```python
from build123d import *

# Parameters (mm, degrees)
SKETCH_1_R               = 39.75
EXTRUDE_1_DEPTH          = 10
SKETCH_2_R               = 18.25
CUT_EXTRUDE_1_DEPTH      = 4
SKETCH_3_R               = 11.5
CUT_EXTRUDE_2_DEPTH      = 2
SKETCH_4_R               = 1.5
CUT_EXTRUDE_3_DEPTH      = 6
SKETCH_5_R               = 3
CUT_EXTRUDE_4_DEPTH      = 2
SKETCH_7_R               = 2.65
CUT_EXTRUDE_5_DEPTH      = 8
PATTERN_CIRCULAR_1_COUNT = 2
PATTERN_CIRCULAR_1_ANGLE = 25
F_1_THE_OTHER_WAY_COUNT  = 2
F_1_THE_OTHER_WAY_ANGLE  = 25
MIRROR_1_COPY_1_SKETCH_R = 2.65
MIRROR_1_COPY_1_DEPTH    = 8
MIRROR_1_COPY_2_SKETCH_R = 2.65
MIRROR_1_COPY_2_DEPTH    = 8
SKETCH_8_R               = 8
CUT_EXTRUDE_6_DEPTH      = 4
SKETCH_9_R               = 2.65
CUT_EXTRUDE_7_DEPTH      = 8
PATTERN_CIRCULAR_2_COUNT = 2
EXTRUDE_START            = 5
SKETCH_10_R              = 23.25
SKETCH_10_R_2            = 18.25
EXTRUDE_2_DEPTH          = 5
CUT_EXTRUDE_START        = -10
CUT_EXTRUDE_8_DEPTH      = 10
FILLET_1_R               = 1


# Read off the part's stored shape, not the designer's step: Вырез-Вытянуть8
with BuildPart() as part:
    # Эскиз1 → Бобышка-Вытянуть1 (new body)
    with BuildSketch(Plane.XY):
        Circle(SKETCH_1_R)
    extrude(amount=EXTRUDE_1_DEPTH)

    # Эскиз2 → Вырез-Вытянуть1 (cut)
    with BuildSketch(Plane.XY.offset(10)):
        Circle(SKETCH_2_R)
    extrude(amount=-CUT_EXTRUDE_1_DEPTH, mode=Mode.SUBTRACT)

    # Эскиз3 → Вырез-Вытянуть2 (cut)
    with BuildSketch(Plane.XY.offset(6)):
        Circle(SKETCH_3_R)
    extrude(amount=-CUT_EXTRUDE_2_DEPTH, mode=Mode.SUBTRACT)

    # Эскиз4 → Вырез-Вытянуть3 (cut)
    with BuildSketch(Plane.XY.offset(6)):
        with Locations((-9.899494937, 9.899494937)):
            Circle(SKETCH_4_R)
        with Locations((9.899494937, 9.899494937)):
            Circle(SKETCH_4_R)
        with Locations((9.899494937, -9.899494937)):
            Circle(SKETCH_4_R)
        with Locations((-9.899494937, -9.899494937)):
            Circle(SKETCH_4_R)
    extrude(amount=-CUT_EXTRUDE_3_DEPTH, mode=Mode.SUBTRACT)

    # Эскиз5 → Вырез-Вытянуть4 (cut)
    with BuildSketch(Plane(origin=(0, 0, 0), x_dir=(-1, 0, 0), z_dir=(0, 0, -1))):
        with Locations((-9.899494937, 9.899494937)):
            Circle(SKETCH_5_R)
        with Locations((9.899494937, 9.899494937)):
            Circle(SKETCH_5_R)
        with Locations((9.899494937, -9.899494937)):
            Circle(SKETCH_5_R)
        with Locations((-9.899494937, -9.899494937)):
            Circle(SKETCH_5_R)
    extrude(amount=-CUT_EXTRUDE_4_DEPTH, mode=Mode.SUBTRACT)

    # Эскиз7 → Вырез-Вытянуть5 (cut)
    with BuildSketch(Plane(origin=(0, 39.75, 0), x_dir=(0, 0, -1), z_dir=(0, 1, 0))):
        with Locations(Location((-5, 0, 0), (0, 0, 90))):
            Circle(SKETCH_7_R)
    cut_extrude_5 = extrude(amount=-CUT_EXTRUDE_5_DEPTH, mode=Mode.SUBTRACT)

    # Круговой массив1: Вырез-Вытянуть5 ×2 about axis
    pattern_circular_1_axis = Axis((0, 0, 10), (0, 0, -1))
    for i in range(1, PATTERN_CIRCULAR_1_COUNT):
        add(cut_extrude_5.rotate(pattern_circular_1_axis, i * PATTERN_CIRCULAR_1_ANGLE / (PATTERN_CIRCULAR_1_COUNT - 1)), mode=Mode.SUBTRACT)

    # 1 the other way: Вырез-Вытянуть5 ×2 about axis
    f_1_the_other_way_axis = Axis((0, 0, 10), (0, 0, 1))
    for i in range(1, F_1_THE_OTHER_WAY_COUNT):
        add(cut_extrude_5.rotate(f_1_the_other_way_axis, i * F_1_THE_OTHER_WAY_ANGLE / (F_1_THE_OTHER_WAY_COUNT - 1)), mode=Mode.SUBTRACT)

    # Зеркальное отражение1: Вырез-Вытянуть5 across plane
    add(cut_extrude_5.mirror(Plane.ZX), mode=Mode.SUBTRACT)

    # Зеркальное отражение1 copy 1 sketch → Зеркальное отражение1 copy 1 (cut)
    with BuildSketch(Plane(origin=(16.799075904, -36.025734535, 0), x_dir=(0, 0, -1), z_dir=(0.4226182617407035, -0.906307787036648, 0))):
        with Locations((-5, 0)):
            Circle(MIRROR_1_COPY_1_SKETCH_R)
    extrude(amount=-MIRROR_1_COPY_1_DEPTH, mode=Mode.SUBTRACT)

    # Зеркальное отражение1 copy 2 sketch → Зеркальное отражение1 copy 2 (cut)
    with BuildSketch(Plane(origin=(-16.799075904, -36.025734535, 0), x_dir=(0, 0, -1), z_dir=(-0.42261826174069717, -0.9063077870366509, 0))):
        with Locations((-5, 0)):
            Circle(MIRROR_1_COPY_2_SKETCH_R)
    extrude(amount=-MIRROR_1_COPY_2_DEPTH, mode=Mode.SUBTRACT)

    # Эскиз8 → Вырез-Вытянуть6 (cut)
    with BuildSketch(Plane.XY.offset(4)):
        Circle(SKETCH_8_R)
    extrude(amount=-CUT_EXTRUDE_6_DEPTH, mode=Mode.SUBTRACT)

    # Эскиз9 → Вырез-Вытянуть7 (cut)
    with BuildSketch(Plane.ZY.offset(39.75)):
        with Locations((5, 0)):
            Circle(SKETCH_9_R)
    cut_extrude_7 = extrude(amount=-CUT_EXTRUDE_7_DEPTH, mode=Mode.SUBTRACT)

    # Круговой массив2: Вырез-Вытянуть7 ×2 about axis
    pattern_circular_2_axis = Axis((0, 0, 10), (0, 0, -1))
    for i in range(1, PATTERN_CIRCULAR_2_COUNT):
        add(cut_extrude_7.rotate(pattern_circular_2_axis, i * 360 / PATTERN_CIRCULAR_2_COUNT), mode=Mode.SUBTRACT)

    # Эскиз10 → Бобышка-Вытянуть2 (add)
    with BuildSketch(Plane.XY.offset(10).offset(EXTRUDE_START)):
        Circle(SKETCH_10_R)
        Circle(SKETCH_10_R_2, mode=Mode.SUBTRACT)
    extrude(amount=-EXTRUDE_2_DEPTH)

    # Вырез-Вытянуть8 outline → Вырез-Вытянуть8 (cut)
    with BuildSketch(Plane(origin=(0, 0, 0), x_dir=(-1, 0, 0), z_dir=(0, 0, -1)).offset(CUT_EXTRUDE_START)):
        with BuildLine():
            Line((36.811173575, 15), (26.811173575, 15))
            Line((26.811173575, 15), (26.811173575, -15))
            Line((26.811173575, -15), (36.811173575, -15))
            ThreePointArc((36.811173575, -15), (39.75, 0), (36.811173575, 15))
        make_face()
    extrude(amount=CUT_EXTRUDE_8_DEPTH, mode=Mode.SUBTRACT)

    # Скругление1
    fillet_1_edges = [part.edges().sort_by_distance(p)[0] for p in [
        (-26.811173575, 15, 5),
        (-26.811173575, -15, 5),
        (-36.811173575, -15, 5),
        (-36.811173575, 15, 5),
    ]]
    fillet(fillet_1_edges, radius=FILLET_1_R)


solid = part.part
```
Part model, mm, in its own coordinate system. A direction names the side the tool comes from. Coordinates: 2 decimals unless noted, no trailing zeros. Write each loop counter-clockwise with the first axis right and the second up, starting at its lowest first coordinate (ties: lowest second). Pieces come first, ordered by that corner, then holes.
Item 1: Probe line 1 (Y direction, x = 0, z = 2.3); line 2 (X direction, y = -9, z = 3.25); line 3 (Y direction, x = -13, z = 6.75). List the from-to ranges inside material, lowest first.
Item 2: Slice it at C-C (z = 11.75). Write the cut outline in (x, y).
Item 3: Slice it at D-D (z = 5). Count the separate pieces of the cut face and the enclosed holes in it, and give its area (3 significant figures).
Item 4: Which spindle directions (+Z, -Z, +X, -X, +Y, -Y) get a long thin tool onto all of the face, cutting with end or side? Do faces 5 (the face through (-11.2, 8.6, 2)), 6 (the face through (-26.811, 0, 5)), 7 (the face through (13.45, 28.76, 5.04)), 8 (the face through (0, -31.75, 5)), 9 (the face through (31.75, 0, 5)). Say none if no direction does.
Item 5: Pin check, flat tips, straight feed: pin 1 (4 mm diameter, centred on x = -18, z = 2.5, fed in from +Y); pin 2 (1.6 mm diameter, centred on x = -0.5, z = 6, fed in from +Y); pin 3 (8 mm diameter, centred on y = -20, z = 9, fed in from +X); pin 4 (1.8 mm diameter, centred on x = 9.5, y = -9.5, fed in from -Z). Stop position of each tip, or through.
Item 6: Mould opens along Y. For faces 1 (the face through (-3.956, -17.816, 10.563)), 2 (the face through (22.176, 6.984, 12.535)), 3 (the face through (0, 31.75, 5)), 4 (the face through (0.57, 35.81, 2.41)) say: released by +Y, released by -Y, zero draft, split by the parting line, or undercut.
Item 7: Slice it at B-B (y = 6). Write the cut outline in (x, z).
Item 8: Slice it at A-A (x = 0). Write the cut outline in (y, z), and give its area (3 significant figures).
Results found:
1. line 1: y = -39.75 to -8, 8 to 39.75
1. line 2: x = -26.81 to -11.1, -8.7 to 8.7, 11.1 to 38.72
1. line 3: y = -37.56 to -32.59, -28.97 to -12.81, 12.81 to 28.97, 32.59 to 37.56
2. outline: circle Ø46.5 at (0, 0); hole circle Ø36.5 at (0, 0)
3. separate pieces: 1
3. enclosed holes: 5
3. area: 3,860 mm2
4. face 5: -Z
4. face 6: +Z, -Z, -X
4. face 7: none
4. face 8: -Y
4. face 9: +X
5. pin 1: stops at y = 36.39
5. pin 2: stops at y = 31.75
5. pin 3: stops at x = 36.39
5. pin 4: passes through
6. face 1: undercut
6. face 2: split by the parting line
6. face 3: released by +Y
6. face 4: zero draft
7. outline: (-26.81, 0) - (-5.29, 0) - (-5.29, 4) - (-9.81, 4) - (-9.81, 6) - (-17.24, 6) - (-17.24, 15) - (-22.46, 15) - (-22.46, 10) - (-26.81, 10) - close; (5.29, 0) - (39.29, 0) - (39.29, 10) - (22.46, 10) - (22.46, 15) - (17.24, 15) - (17.24, 6) - (9.81, 6) - (9.81, 4) - (5.29, 4) - close
8. outline: (-39.75, 0) - (-8, 0) - (-8, 4) - (-11.5, 4) - (-11.5, 6) - (-18.25, 6) - (-18.25, 15) - (-23.25, 15) - (-23.25, 10) - (-39.75, 10) - (-39.75, 7.65) - (-31.75, 7.65) - (-31.75, 2.35) - (-39.75, 2.35) - close; (8, 0) - (39.75, 0) - (39.75, 2.35) - (31.75, 2.35) - (31.75, 7.65) - (39.75, 7.65) - (39.75, 10) - (23.25, 10) - (23.25, 15) - (18.25, 15) - (18.25, 6) - (11.5, 6) - (11.5, 4) - (8, 4) - close
8. area: 504 mm2
